Source: CAD feature listing. Evaluate the final solid. Frame: model axes, mm. A direction names the side the tool comes from. Give positions to 0.01 mm unless a question says otherwise; leave off trailing zeros. Order: outer loops, then holes, each group sorted by start corner. A loop starts at its lowest first (then second) coordinate and runs counter-clockwise, first axis right, second up.
```python
from build123d import *

# Parameters (mm, degrees)
F0_R     = 8
F1_DEPTH = 3.5
F2_DEPTH = 1
F3_W     = 20
F3_H     = 2
F4_DEPTH = 2


with BuildPart() as f1:
    # F0 (on Top) → F1 (new body)
    with BuildSketch(Plane.XY):
        with BuildLine():
            ThreePointArc((0, -12.5), (8.838835, -8.838835), (12.5, 0))
            ThreePointArc((12.5, 0), (8.838835, 8.838835), (0, 12.5))
            ThreePointArc((0, 12.5), (-12.5, 0), (0, -12.5))
        make_face()
        Circle(F0_R, mode=Mode.SUBTRACT)
        with BuildLine():
            ThreePointArc((0, -12.5), (-12.5, 0), (0, 12.5))
            Line((0, 12.5), (-35, 12.5))
            Line((-35, 12.5), (-116.388784, 2.506714))
            Line((-116.388784, 2.506714), (-116.388784, -2.506714))
            Line((-116.388784, -2.506714), (-35, -12.5))
            Line((-35, -12.5), (0, -12.5))
        make_face()
    extrude(amount=F1_DEPTH)

    # F0 (on Top) → F2 (join)
    with BuildSketch(Plane.XY):
        Circle(F0_R)
    extrude(amount=F2_DEPTH)

    # F3 (on face) → F4 (cut)
    with BuildSketch(Plane.XY.offset(3.5)):
        with Locations((-106.388784, 0.006714)):
            Rectangle(F3_W, F3_H)
    extrude(amount=-F4_DEPTH, mode=Mode.SUBTRACT)


solid = f1.part
```
1) Section query C-C, the plane x = -45. Return the cut outline in (y, z), and give its area (3 significant figures).
Report:
outline: (-11.27, 0) - (11.27, 0) - (11.27, 3.5) - (-11.27, 3.5) - close
area: 78.9 mm2
2) Section query A-A, the plane z = 2.25. Return the cut outline in (x, y).
Report:
outline: (-116.39, -2.51) - (-35, -12.5) - (0, -12.5) arc R12.5 ccw to (12.5, 0) arc R12.5 ccw to (0, 12.5) - (-35, 12.5) - (-116.39, 2.51) - (-116.39, 1.01) - (-96.39, 1.01) - (-96.39, -0.99) - (-116.39, -0.99) - close; hole circle Ø16 at (0, 0)
3) Section query B-B, the plane y = 9.5. Return the cut outline in (x, z), and give its area (3 significant figures).
Report:
outline: (-59.43, 0) - (8.12, 0) - (8.12, 3.5) - (-59.43, 3.5) - close
area: 236 mm2
4) Pin query (flat end, axial travel): pin 1 (0.6 mm diameter, centred on x = -110.5, z = 2.5, fed in from -Y); pin 2 (5 mm diameter, centred on x = 0.5, y = -1, fed in from +Z); pin 3 (2 mm diameter, centred on x = -104.5, z = 2.5, fed in from +Y). Return the tip coordinate at first contact, or that it passes through.
Report:
pin 1: stops at y = -3.27
pin 2: stops at z = 1
pin 3: stops at y = 4.09
5) Draft query along Y for faces 4 (the flat face through (-75.125, 7.573, 1.726)), 5 (the flat face through (-107, -0.993, 3)), 6 (the flat face through (-39, 0, 0)). Return one class per face: +Y half, -Y half, draft (parallel to the pull), parting line (faces both ways), or undercut.
Report:
face 4: +Y half
face 5: undercut
face 6: draft
6) Material intervals for L1, parallel to Y at x = 0, z = 2.35; L2, parallel to X at y = -0.5, z = 0.7; L3, parallel to X at y = 0.25, z = 2.1, sorted ascending.
Report:
L1: y = -12.5 to -8, 8 to 12.5
L2: x = -116.39 to 12.49
L3: x = -96.39 to -8, 8 to 12.5
7) Reachability of faces 1 (the flat face through (-18, -12.5, 2)), 2 (the cylindrical face through (-1.73, -7.81, 2.23)), 3 (the flat face through (-96.389, 0, 3)) from +Z, -Z, +X, -X, +Y, -Y: full face, straight path, thin tool, end or side. Return the list, or none.
Report:
face 1: +Z, -Z, +X, -X, -Y
face 2: +Z
face 3: +Z, -X
